Part model, mm, in its own coordinate system. A direction names the side the tool comes from. Round coordinates to 2 decimals unless told otherwise and drop trailing zeros. Write each loop counter-clockwise with the first axis right and the second up, starting at its lowest first coordinate (ties: lowest second). Pieces come first, ordered by that corner, then holes. Notation, with made-up numbers: (71, 42) -> (99, 42) arc R30 ccw to (99, 76) -> close; hole circle Ø5 at (46, -3). An arc over 180 degrees is marked (long way). Return JSON: item names as keys, results as strings. Group by question number.
(1) Saw through at A-A (z = 0). List the corners of the cut face in (x, y), plus the area to 3 significant figures.
(2) Mould opens along Z. For faces 3 (the flat face through (-13, 14, -1)), 4 (the cylindrical face through (2.75, 6.9, -62.44)), 5 (the cylindrical face through (14.215, 7.409, -12.002)) say: +Z half, -Z half, draft (parallel to the pull), parting line (faces both ways), or undercut.
(3) Saw through at B-B (x = 0). List the corners of the cut face in (y, z).
(4) Drill centre lines: L1, parallel to X at y = 8.25, z = 0; L2, parallel to Z at x = 9, y = 4; L3, parallel to Z at x = 15, y = 12.25. Where is each one in solid material? Low to high. Write a range as from..to.
(5) Saw through at C-C (y = 11.75). List the corners of the cut face in (x, z), plus the area to 3 significant figures.
(6) Saw through at D-D (x = -17). List the corners of the cut face in (y, z), plus the area to 3 significant figures.
(7) Tool access for faces 1 (the flat face through (-13, 0, -1)), 2 (the flat face through (11, 1, -19)): list every direction of +Z, -Z, +X, -X, +Y, -Y with a clear straight run to the whole face (end or side of a thin tool).
(8) Drop flat-ended pins along their axis: pin 1 Ø1.5 at (y, z) = (3.5, -15.5) entering from -X; pin 2 Ø2 at (x, y) = (38, 3) entering from -Z; pin 3 Ø1.5 at (x, y) = (25.5, 2.5) entering from +Z. Give the stop position or say it passes through.
from build123d import *

# Parameters (mm, degrees)
SKETCH1_R             = 62.5
BOSS_EXTRUDE1_DEPTH   = 14
SKETCH2_R             = 7.5
CUT_EXTRUDE1_DEPTH    = 90.49022293
SKETCH3_R             = 7.483126217
CUT_EXTRUDE2_DEPTH    = 13.000434
CIRPATTERN1_START     = 0.999566119
CIRPATTERN1_OUTLINE_R = 7.483126217
CIRPATTERN1_DEPTH     = 13.000433881


# Read off the part's stored shape, not the designer's step: CirPattern1
with BuildPart() as part:
    # Sketch1 → Boss-Extrude1 (new body)
    with BuildSketch(Plane(origin=(0, 0, 0), x_dir=(1, 0, 0), z_dir=(0, 1, 0))):
        with Locations(Location((0, 0, 0), (0, 0, 270))):
            Circle(SKETCH1_R)
    extrude(amount=BOSS_EXTRUDE1_DEPTH)

    # Sketch2 → Cut-Extrude1 (cut, through all)
    with BuildSketch(Plane(origin=(0, 0, 0), x_dir=(1, 0, 0), z_dir=(0, 1, 0))):
        with Locations(Location((0, 0, 0), (0, 0, 270))):
            Circle(SKETCH2_R)
    extrude(amount=CUT_EXTRUDE1_DEPTH, mode=Mode.SUBTRACT)

    # Sketch3 → Cut-Extrude2 (cut)
    with BuildSketch(Plane(origin=(0, 14, 0), x_dir=(1, 0, 0), z_dir=(0, 1, 0))):
        with Locations(Location((-21.524422903, 0, 0), (0, 0, 270))):
            Circle(SKETCH3_R)
    extrude(amount=-CUT_EXTRUDE2_DEPTH, mode=Mode.SUBTRACT)

    # CirPattern1 outline → CirPattern1 (cut)
    with BuildSketch(Plane(origin=(0, 0, 0), x_dir=(1, 0, 0), z_dir=(0, 1, 0)).offset(CIRPATTERN1_START)):
        with Locations((10.762211451, 18.640697036)):
            Circle(CIRPATTERN1_OUTLINE_R)
        with Locations((10.762211451, -18.640697036)):
            Circle(CIRPATTERN1_OUTLINE_R)
    extrude(amount=CIRPATTERN1_DEPTH, mode=Mode.SUBTRACT)


solid = part.part
Computed values:
{
 "1": {"outline": "(-62.5, 0) -> (-7.5, 0) -> (-7.5, 14) -> (-14.04, 14) -> (-14.04, 1) -> (-29.01, 1) -> (-29.01, 14) -> (-62.5, 14) -> close; (7.5, 0) -> (62.5, 0) -> (62.5, 14) -> (7.5, 14) -> close", "area": "1,350 mm2"},
 "2": {"face 3": "draft", "face 4": "parting line", "face 5": "undercut"},
 "3": {"outline": "(0, -62.5) -> (14, -62.5) -> (14, -7.5) -> (0, -7.5) -> close; (0, 7.5) -> (14, 7.5) -> (14, 62.5) -> (0, 62.5) -> close"},
 "4": {"L1": "-62.5..-29.01, -14.04..-7.5, 7.5..62.5", "L2": "-61.85..-25.91, -11.37..11.37, 25.91..61.85", "L3": "-60.67..-24.81, -12.47..12.47, 24.81..60.67"},
 "5": {"outline": "circle Ø125 at (0, 0); hole circle Ø14.97 at (-21.52, 0); hole circle Ø15 at (0, 0); hole circle Ø14.97 at (10.76, -18.64); hole circle Ø14.97 at (10.76, 18.64)", "area": "11,600 mm2"},
 "6": {"outline": "(0, -60.14) -> (14, -60.14) -> (14, -5.96) -> (1, -5.96) -> (1, 5.96) -> (14, 5.96) -> (14, 60.14) -> (0, 60.14) -> close", "area": "1,530 mm2"},
 "7": {"face 1": "+Z, -Z, +X, -X, -Y", "face 2": "+Y"},
 "8": {"pin 1": "x = -60.73", "pin 2": "z = -50.37", "pin 3": "z = 57.39"}
}
